from build123d import *

# Parameters (mm, degrees)
ESQUISSE1_R        = 5.406629484
ESQUISSE1_R_2      = 5.395392345
ESQUISSE1_R_3      = 4.854658012
ESQUISSE1_R_4      = 4.85477379
BOSS_EXTRU_1_DEPTH = 5
CONG_1_R           = 10


with BuildPart() as part:
    # Esquisse1 → Boss.-Extru.1 (new body)
    with BuildSketch(Plane.XY):
        with BuildLine():
            Line((-10, 0), (-12, 0))
            ThreePointArc((-12, 0), (-9.447374533, 49.977092468), (-27.5, 96.649658093))
            Line((-27.5, 96.649658093), (-27.5, 101.649658093))
            Line((-27.5, 101.649658093), (-22.5, 101.649658093))
            Line((-22.5, 101.649658093), (-22.5, 106.649658093))
            Line((-22.5, 106.649658093), (-17.5, 106.649658093))
            Line((-17.5, 106.649658093), (-17.5, 101.649658093))
            Line((-17.5, 101.649658093), (-14, 101.649658093))
            Line((-14, 101.649658093), (-14, 98.649658093))
            Line((-14, 98.649658093), (-15.1, 98.649658093))
            Line((-15.1, 98.649658093), (-15.1, 96.349658093))
            Line((-15.1, 96.349658093), (-14, 96.349658093))
            Line((-14, 96.349658093), (-14, 91.649658093))
            Line((-14, 91.649658093), (-11, 91.649658093))
            Line((-11, 91.649658093), (-11, 96.349658093))
            Line((-11, 96.349658093), (-9.9, 96.349658093))
            Line((-9.9, 96.349658093), (-9.9, 98.649658093))
            Line((-9.9, 98.649658093), (-11, 98.649658093))
            Line((-11, 98.649658093), (-11, 101.649658093))
            Line((-11, 101.649658093), (-7.5, 101.649658093))
            Line((-7.5, 101.649658093), (-7.5, 106.649658093))
            Line((-7.5, 106.649658093), (-2.5, 106.649658093))
            Line((-2.5, 106.649658093), (-2.5, 101.649658093))
            Line((-2.5, 101.649658093), (2.5, 101.649658093))
            Line((2.5, 101.649658093), (2.5, 106.649658093))
            Line((2.5, 106.649658093), (7.5, 106.649658093))
            Line((7.5, 106.649658093), (7.5, 101.649658093))
            Line((7.5, 101.649658093), (11, 101.649658093))
            Line((11, 101.649658093), (11, 98.649658093))
            Line((11, 98.649658093), (9.9, 98.649658093))
            Line((9.9, 98.649658093), (9.9, 96.349658093))
            Line((9.9, 96.349658093), (11, 96.349658093))
            Line((11, 96.349658093), (11, 91.649658093))
            Line((11, 91.649658093), (14, 91.649658093))
            Line((14, 91.649658093), (14, 96.349658093))
            Line((14, 96.349658093), (15.1, 96.349658093))
            Line((15.1, 96.349658093), (15.1, 98.649658093))
            Line((15.1, 98.649658093), (14, 98.649658093))
            Line((14, 98.649658093), (14, 101.649658093))
            Line((14, 101.649658093), (17.5, 101.649658093))
            Line((17.5, 101.649658093), (17.5, 106.649658093))
            Line((17.5, 106.649658093), (22.5, 106.649658093))
            Line((22.5, 106.649658093), (22.5, 101.649658093))
            Line((22.5, 101.649658093), (27.5, 101.649658093))
            Line((27.5, 101.649658093), (27.5, 96.649658093))
            ThreePointArc((27.5, 96.649658093), (9.447374533, 49.977092468), (12, 0))
            Line((12, 0), (10, 0))
            Line((10, 0), (10, -5))
            Line((10, -5), (5, -5))
            Line((5, -5), (5, 0))
            Line((5, 0), (1.5, 0))
            Line((1.5, 0), (1.5, 3))
            Line((1.5, 3), (2.6, 3))
            Line((2.6, 3), (2.6, 5.3))
            Line((2.6, 5.3), (1.5, 5.3))
            Line((1.5, 5.3), (1.5, 10))
            Line((1.5, 10), (-1.5, 10))
            Line((-1.5, 10), (-1.5, 5.3))
            Line((-1.5, 5.3), (-2.6, 5.3))
            Line((-2.6, 5.3), (-2.6, 3))
            Line((-2.6, 3), (-1.5, 3))
            Line((-1.5, 3), (-1.5, 0))
            Line((-1.5, 0), (-5, 0))
            Line((-5, 0), (-5, -5))
            Line((-5, -5), (-10, -5))
            Line((-10, -5), (-10, 0))
        make_face()
        with Locations((7.512942396, 82.788090233)):
            Circle(ESQUISSE1_R, mode=Mode.SUBTRACT)
        with Locations((-4.245332426, 69.827264576)):
            Circle(ESQUISSE1_R_2, mode=Mode.SUBTRACT)
        with Locations((1.500188226, 50.051984193)):
            Circle(ESQUISSE1_R_3, mode=Mode.SUBTRACT)
        with Locations((0, 26.401817788)):
            Circle(ESQUISSE1_R_4, mode=Mode.SUBTRACT)
    extrude(amount=BOSS_EXTRU_1_DEPTH)

    # Congé1
    cong_1_edges = [part.edges().sort_by_distance(p)[0] for p in [
        (27.5, 96.649658093, 2.5),
        (-27.5, 96.649658093, 2.5),
    ]]
    fillet(cong_1_edges, radius=CONG_1_R)


solid = part.part
Read the model definition and answer for the solid it produces. Units are mm, in the model's axes. A direction names the side the tool comes from. Round coordinates to 2 decimals unless told otherwise and drop trailing zeros. Write each loop counter-clockwise with the first axis right and the second up, starting at its lowest first coordinate (ties: lowest second). Pieces come first, ordered by that corner, then holes. Notation, with made-up numbers: (-18, 59) - (3, 59) arc R23 ccw to (3, 83) - close; hole circle Ø10 at (59.5, -20.75). An arc over 180 degrees is marked (long way). Use a Markdown table: item, result.
(1) The part is cut by section D-D (y = 42). Write down the section's boundary in (x, z), then the cut area to 3 significant figures.
Reported:
| item | result |
|---|---|
| outline | (-8.44, 0) - (8.44, 0) - (8.44, 5) - (-8.44, 5) - close |
| area | 84.4 mm2 |
(2) Each of these flat-tipped pins is pushed along its axis until it touches: pin 1 Ø2.5 at (y, z) = (95, 2.5) entering from +X; pin 2 Ø1.5 at (x, z) = (12, 3) entering from +Y; pin 3 Ø1.2 at (x, z) = (14.5, 3.5) entering from +Y. Where does it stop, or does it pass through?
Reported:
| item | result |
|---|---|
| pin 1 | x = 26.93 |
| pin 2 | y = 91.65 |
| pin 3 | y = 101.65 |
(3) Straight lines are drawn through the part: line 1 along X through (y, z) = (4, 3.9); line 2 along X through (y, z) = (95, 0.85); line 3 along Y through (x, z) = (0, 4.3). For each, find the intervals that lie inside material, in ascending order. Write a range as [from, to].
Reported:
| item | result |
|---|---|
| line 1 | [-11, -2.6], [2.6, 11] |
| line 2 | [-26.4, -14], [-11, 11], [14, 26.4] |
| line 3 | [10, 21.55], [31.26, 45.43], [54.67, 66.5], [73.16, 101.65] |
(4) The mould has two halves that part along X. Classify faces 1 (the flat face through (25, 101.65, 2)), 2 (the flat face through (-27.5, 101, 2)), 3 (the flat face through (12, 91.65, 2)), 4 (the flat face through (2.6, 4, 2)): released by +X, released by -X, zero draft, split by the parting line, or undercut.
Reported:
| item | result |
|---|---|
| face 1 | zero draft |
| face 2 | released by -X |
| face 3 | undercut |
| face 4 | undercut |
(5) Which of the six approach directions +Z, -Z, +X, -X, +Y, -Y give full straight-line access (tool end or side, diameter ignored) to faces 5 (the flat face through (-25, 101.65, 2)), 6 (the flat face through (-13, 91.65, 2)), 7 (the flat face through (15.1, 97, 2))?
Reported:
| item | result |
|---|---|
| face 5 | +Z, -Z, -X, +Y |
| face 6 | +Z, -Z, +Y |
| face 7 | +Z, -Z |
(6) The part is cut by section C-C (z = 3.2). State how many separate pieces and enclosed holes the cut face has, then the cut area to 3 significant figures.
Reported:
| item | result |
|---|---|
| separate pieces | 1 |
| enclosed holes | 4 |
| area | 2,430 mm2 |
(7) The part is cut by section A-A (y = 87). Write down the section's boundary in (x, z), then the cut area to 3 significant figures.
Reported:
| item | result |
|---|---|
| outline | (-21.81, 0) - (4.12, 0) - (4.12, 5) - (-21.81, 5) - close; (10.9, 0) - (21.81, 0) - (21.81, 5) - (10.9, 5) - close |
| area | 184 mm2 |
(8) The part is cut by section B-B (x = 0). Write down the section's boundary in (y, z), then the cut area to 3 significant figures.
Reported:
| item | result |
|---|---|
| outline | (10, 0) - (21.55, 0) - (21.55, 5) - (10, 5) - close; (31.26, 0) - (45.43, 0) - (45.43, 5) - (31.26, 5) - close; (54.67, 0) - (66.5, 0) - (66.5, 5) - (54.67, 5) - close; (73.16, 0) - (101.65, 0) - (101.65, 5) - (73.16, 5) - close |
| area | 330 mm2 |
